```python
from build123d import *

# Parameters (mm, degrees)
SKETCH2_W                                       = 134
SKETCH2_H                                       = 104
BOSS_EXTRUDE1_DEPTH                             = 10
SKETCH3_W                                       = 7.2
SKETCH3_H                                       = 23
BOSS_EXTRUDE2_DEPTH                             = 7.9
BOSS_EXTRUDE3_DEPTH                             = 7.9
CSK_FOR_M4_FLAT_HEAD_MACHINE_SCREW1_D           = 4.5
CSK_FOR_M4_FLAT_HEAD_MACHINE_SCREW1_DEPTH       = 10
CSK_FOR_M4_FLAT_HEAD_MACHINE_SCREW1_CSINK_D     = 9.4
CSK_FOR_M4_FLAT_HEAD_MACHINE_SCREW1_CSINK_ANGLE = 90
CSK_FOR_M4_FLAT_HEAD_MACHINE_SCREW1_TIP         = 1.351936393
SKETCH4_R                                       = 2.4
CUT_EXTRUDE3_DEPTH                              = 124.303600725
SKETCH8_W                                       = 20
SKETCH8_H                                       = 32
BOSS_EXTRUDE4_DEPTH                             = 32
CSK_FOR_M3_FLAT_HEAD_MACHINE_SCREW1_D           = 3.4
CSK_FOR_M3_FLAT_HEAD_MACHINE_SCREW1_DEPTH       = 10
CSK_FOR_M3_FLAT_HEAD_MACHINE_SCREW1_CSINK_D     = 6.3
CSK_FOR_M3_FLAT_HEAD_MACHINE_SCREW1_CSINK_ANGLE = 90
CSK_FOR_M3_FLAT_HEAD_MACHINE_SCREW1_TIP         = 1.021463052
CSK_FOR_M4_FLAT_HEAD_MACHINE_SCREW2_D           = 4.5
CSK_FOR_M4_FLAT_HEAD_MACHINE_SCREW2_CSINK_D     = 9.4
CSK_FOR_M4_FLAT_HEAD_MACHINE_SCREW2_CSINK_ANGLE = 90
SKETCH9_W                                       = 48.824666317
SKETCH9_H                                       = 29.759338586
CUT_EXTRUDE4_DEPTH                              = 11


with BuildPart() as part:
    # Sketch2 → Boss-Extrude1 (new body)
    with BuildSketch(Plane(origin=(0, 0, 0), x_dir=(1, 0, 0), z_dir=(0, 1, 0))):
        with Locations((4.53434515, -5.431597684)):
            Rectangle(SKETCH2_W, SKETCH2_H)
    extrude(amount=BOSS_EXTRUDE1_DEPTH)

    # Sketch3 → Boss-Extrude2 (add)
    with BuildSketch(Plane(origin=(0, 10, 0), x_dir=(1, 0, 0), z_dir=(0, 1, 0))):
        with Locations((-48.169255575, -4.929066507)):
            Rectangle(SKETCH3_W, SKETCH3_H)
        with Locations((-32.22922018, -4.929066507)):
            Rectangle(SKETCH3_W, SKETCH3_H)
        with Locations((-16.128962561, -4.929066507)):
            Rectangle(SKETCH3_W, SKETCH3_H)
    extrude(amount=BOSS_EXTRUDE2_DEPTH)

    # Sketch5 → Boss-Extrude3 (add)
    with BuildSketch(Plane(origin=(0, 10, 0), x_dir=(1, 0, 0), z_dir=(0, 1, 0))):
        Polygon((-20.32922018, -42.887289811), (-20.32922018, -23.319494658), (-44.195608335, -23.319494658), (-44.100155676, -42.887289811), align=None)
    extrude(amount=BOSS_EXTRUDE3_DEPTH)

    # CSK for M4 Flat Head Machine Screw1
    with Locations(Plane(origin=(0, 10, 0), x_dir=(1, 0, 0), z_dir=(0, 1, 0))):
        with Locations((-57.46565485, 40.568402316), (-33.46565485, 40.568402316), (-57.46565485, 22.568402316), (-33.46565485, 22.568402316), (-57.46565485, -33.431597684), (-57.46565485, -51.431597684), (-33.46565485, -51.431597684), (42.53434515, -33.431597684), (66.53434515, -33.431597684), (42.53434515, -51.431597684), (66.53434515, -51.431597684), (42.53434515, 40.568402316), (66.53434515, 40.568402316), (66.53434515, 22.568402316), (42.53434515, 22.568402316)):
            CounterSinkHole(CSK_FOR_M4_FLAT_HEAD_MACHINE_SCREW1_D / 2, CSK_FOR_M4_FLAT_HEAD_MACHINE_SCREW1_CSINK_D / 2, depth=CSK_FOR_M4_FLAT_HEAD_MACHINE_SCREW1_DEPTH, counter_sink_angle=CSK_FOR_M4_FLAT_HEAD_MACHINE_SCREW1_CSINK_ANGLE)
            with Locations((0, 0, -(CSK_FOR_M4_FLAT_HEAD_MACHINE_SCREW1_DEPTH + CSK_FOR_M4_FLAT_HEAD_MACHINE_SCREW1_TIP / 2))):  # 118° drill point
                Cone(0, CSK_FOR_M4_FLAT_HEAD_MACHINE_SCREW1_D / 2, CSK_FOR_M4_FLAT_HEAD_MACHINE_SCREW1_TIP, mode=Mode.SUBTRACT)

    # Sketch4 → Cut-Extrude3 (cut, through all)
    with BuildSketch(Plane.ZY.offset(51.769255575)):
        with Locations((12.929066507, 13.7)):
            Circle(SKETCH4_R)
        with Locations((4.929066507, 13.7)):
            Circle(SKETCH4_R)
        with Locations((-3.070933493, 13.7)):
            Circle(SKETCH4_R)
    extrude(amount=-CUT_EXTRUDE3_DEPTH, mode=Mode.SUBTRACT)

    # Sketch8 → Boss-Extrude4 (add)
    with BuildSketch(Plane(origin=(0, 10, 0), x_dir=(1, 0, 0), z_dir=(0, 1, 0))):
        with Locations((61.53434515, -5.431597684)):
            Rectangle(SKETCH8_W, SKETCH8_H)
    extrude(amount=BOSS_EXTRUDE4_DEPTH)

    # CSK for M3 Flat Head Machine Screw1
    with Locations(Plane(origin=(71.53434515, 0, 0), x_dir=(0, 0, -1), z_dir=(1, 0, 0))):
        with Locations((-17.431597684, 34.83), (-9.931597684, 34.83), (-0.931597684, 34.83), (6.568402316, 34.83)):
            CounterSinkHole(CSK_FOR_M3_FLAT_HEAD_MACHINE_SCREW1_D / 2, CSK_FOR_M3_FLAT_HEAD_MACHINE_SCREW1_CSINK_D / 2, depth=CSK_FOR_M3_FLAT_HEAD_MACHINE_SCREW1_DEPTH, counter_sink_angle=CSK_FOR_M3_FLAT_HEAD_MACHINE_SCREW1_CSINK_ANGLE)
            with Locations((0, 0, -(CSK_FOR_M3_FLAT_HEAD_MACHINE_SCREW1_DEPTH + CSK_FOR_M3_FLAT_HEAD_MACHINE_SCREW1_TIP / 2))):  # 118° drill point
                Cone(0, CSK_FOR_M3_FLAT_HEAD_MACHINE_SCREW1_D / 2, CSK_FOR_M3_FLAT_HEAD_MACHINE_SCREW1_TIP, mode=Mode.SUBTRACT)

    # CSK for M4 Flat Head Machine Screw2 (through all)
    with Locations(Plane(origin=(0, 17.9, 0), x_dir=(1, 0, 0), z_dir=(0, 1, 0))):
        with Locations((-33.46565485, -33.431597684)):
            CounterSinkHole(CSK_FOR_M4_FLAT_HEAD_MACHINE_SCREW2_D / 2, CSK_FOR_M4_FLAT_HEAD_MACHINE_SCREW2_CSINK_D / 2, counter_sink_angle=CSK_FOR_M4_FLAT_HEAD_MACHINE_SCREW2_CSINK_ANGLE)

    # Sketch9 → Cut-Extrude4 (cut, through all)
    with BuildSketch(Plane(origin=(0, 10, 0), x_dir=(1, 0, 0), z_dir=(0, 1, 0))):
        with Locations((2.204099142, 26.778317221)):
            Rectangle(SKETCH9_W, SKETCH9_H)
    extrude(amount=-CUT_EXTRUDE4_DEPTH, mode=Mode.SUBTRACT)


solid = part.part
```
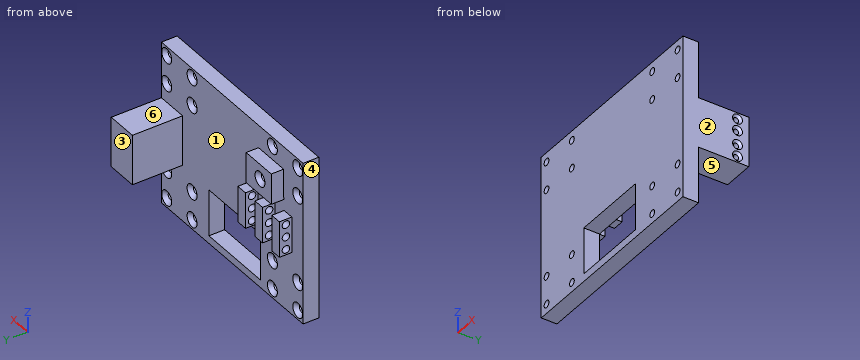
Verification items for the finished model (mm, model axes). Face numbers are marked on the shaded views. A direction names the side the tool comes from. Round coordinates to 2 decimals unless told otherwise and drop trailing zeros. Write each loop counter-clockwise with the first axis right and the second up, starting at its lowest first coordinate (ties: lowest second). Pieces come first, ordered by that corner, then holes. Notation, with made-up numbers: (36.25, 28) -> (70.25, 28) arc R24 cw to (70.25, 43) -> close; hole circle Ø4 at (39, 18). An arc over 180 degrees is marked (long way). Write each question's results on one line, items separated by ' | '. Start each with the question number.
1. Cross-section at B-B (y = 13.7). Count the separate pieces of the cut face and the enclosed holes in it, then the cut area to 3 significant figures.
2. Material ranges on probe 1 along Y at (x, z) = (-45, 29.5); probe 2 along Z at (x, y) = (53.5, 36.5); probe 3 along Y at (x, z) = (-51.5, 11), recorded low to high. Write a range as from..to.
3. Cross-section at A-A (x = -6). Enter the section's corners in (y, z).
4. Cross-section at D-D (y = 22). Enter the section's corners in (x, z), then the cut area to 3 significant figures.
5. Draft check along X on the marked faces 1, 2 and 3. Enter one of: +X half, -X half, draft (parallel to the pull), parting line (faces both ways), or undercut.
6. Set-up check for the marked faces 4, 5 and 6: record each of +Z, -Z, +X, -X, +Y, -Y from which the full face is reachable in a straight line by a thin tool's end or side.
7. Depth check by flat-ended pin: P1, Ø4, axis at y = 12.5, z = 6.5, coming from the -X side; P2, Ø4, axis at y = 15, z = 36.5, coming from the +X side; P3, Ø3, axis at y = 13.7, z = -3.07, coming from the -X side. Enter the tip coordinate at first touch or a pass-through.
Solutions:
1) separate pieces: 14 | enclosed holes: 1 | area: 1,280 mm2
2) probe 1: y = 0..10 | probe 2: z = -10.57..21.43 | probe 3: y = 0..12.27, 15.13..17.9
3) outline: (0, -46.57) -> (10, -46.57) -> (10, -41.66) -> (0, -41.66) -> close; (0, -11.9) -> (10, -11.9) -> (10, 57.43) -> (0, 57.43) -> close
4) outline: (51.53, -10.57) -> (71.53, -10.57) -> (71.53, 21.43) -> (51.53, 21.43) -> close | area: 640 mm2
5) face 1: undercut | face 2: +X half | face 3: draft
6) face 4: +Z, -Z, -X, +Y, -Y | face 5: -Z, +X, -X, +Y | face 6: +Z, +X, -X, +Y
7) P1: stops at x = -51.77 | P2: stops at x = -20.33 | P3: stops at x = 51.53
